```python
from build123d import *

# Parameters (mm, degrees)
CYLINDER062_R     = 1
CYLINDER062_DEPTH = 20
CYLINDER063_R     = 1
CYLINDER063_DEPTH = 20
CYLINDER067_R     = 2.6
CYLINDER067_DEPTH = 12
CYLINDER068_R     = 7
CYLINDER068_DEPTH = 6


with BuildPart() as obj1:
    # Cylinder062 → Cylinder062 (new body)
    with BuildSketch(Plane(origin=(-3.5, -3.5, 0), x_dir=(1, 0, 0), z_dir=(0, 0, 1))):
        Circle(CYLINDER062_R)
    extrude(amount=CYLINDER062_DEPTH)


with BuildPart() as compound034:
    # Cylinder063 → Cylinder063 (new body)
    with BuildSketch(Plane(origin=(3.5, 3.5, 0), x_dir=(1, 0, 0), z_dir=(0, 0, 1))):
        Circle(CYLINDER063_R)
    extrude(amount=CYLINDER063_DEPTH)

    # Compound034: union obj1
    add(obj1.part)


with BuildPart() as obj2:
    # Cylinder067 → Cylinder067 (new body)
    with BuildSketch(Plane.XY.offset(13)):
        Circle(CYLINDER067_R)
    extrude(amount=CYLINDER067_DEPTH)


with BuildPart() as cut037:
    # Cylinder068 → Cylinder068 (new body)
    with BuildSketch(Plane.XY.offset(13)):
        Circle(CYLINDER068_R)
    extrude(amount=CYLINDER068_DEPTH)

    # Cut036: cut obj2
    add(obj2.part, mode=Mode.SUBTRACT)


with BuildPart() as cut037_1:
    # Cut036 placement: moved
    add(cut037.part.moved(Location((0, 0, -2))))

    # Cut037: cut Compound034
    add(compound034.part, mode=Mode.SUBTRACT)


solid = cut037_1.part
```
Can you work these out from the model? Positions are in its coordinate system, mm. Coordinates: 2 decimals unless noted, no trailing zeros. Loops run counter-clockwise (first coordinate to the right, second up) from the corner with the lowest first, then second, coordinate; pieces in that order, holes last. Notation, with made-up numbers: (78, -23) - (114, -23) arc R22 ccw to (114, 13) - close; hole circle Ø8 at (-40, 83). An arc over 180 degrees is marked (long way). Answer as CSV lines item,"result". Start each with the question number.
1) For pin 1 (2 mm diameter, centred on y = 3, z = 15, fed in from -X), with a flat end and sliding along its axis, tell me the tip position at first contact or that it passes through.
2) Thinking about a two-plate mould opening in X: for faces 1 (the cylindrical face through (2.763, 4.176, 13.958)), 2 (the cylindrical face through (6.466, -2.681, 13.958)), 3 (the flat face through (0, -3, 11)), which applies, pulls with the +X half, pulls with the -X half, needs draft (parallel to the pull), parting line crosses it, or undercut?
3) I need wall thicknesses on line 1 (Y direction, x = 0, z = 15.25); line 2 (Y direction, x = -4.25, z = 12.1); line 3 (X direction, y = -3.5, z = 12.3). Which ranges of each line are inside material? Lowest first, please. Write a range as from..to.
4) Suppose I cut it at C-C (z = 14.6). Please give me the cut outline in (x, y), plus the area to 3 significant figures.
5) Suppose I cut it at A-A (y = 0). Please give me the cut outline in (x, z), plus the area to 3 significant figures.
Check result:
1,pin 1,"stops at x = -6.71"
2,face 1,"undercut"
2,face 2,"parting line crosses it"
2,face 3,"needs draft"
3,line 1,"y = -7..-2.6, 2.6..7"
3,line 2,"y = -5.56..-4.16, -2.84..5.56"
3,line 3,"x = -6.06..-4.5, -2.5..6.06"
4,outline,"circle Ø14 at (0, 0); hole circle Ø2 at (-3.5, -3.5); hole circle Ø5.2 at (0, 0); hole circle Ø2 at (3.5, 3.5)"
4,area,"126 mm²"
5,outline,"(-7, 11) - (-2.6, 11) - (-2.6, 17) - (-7, 17) - close; (2.6, 11) - (7, 11) - (7, 17) - (2.6, 17) - close"
5,area,"52.8 mm²"
